```python
from build123d import *

# Parameters (mm, degrees)
F0_R      = 38.279248166
F2_R      = 18.7324901921
F5_R      = 38.2461043671
F3_FACE_R = 18.7324901921
F7_T      = -2.5


with BuildPart() as f3:
    # F0 (on Front) → F3 section 0
    with BuildSketch(Plane.XZ):
        Circle(F0_R)
    # F2 (on offset) → F3 section 1
    with BuildSketch(Plane.XZ.offset(100)):
        Circle(F2_R)
    loft()

    # F5 (on offset) → F6 section 0
    with BuildSketch(Plane.XZ.offset(200)):
        Circle(F5_R)
    # F3_face (on face) → F6 section 1
    with BuildSketch(Plane.XZ.offset(100)):
        Circle(F3_FACE_R)
    loft()

    # F7
    f7_openings = [f3.faces().sort_by_distance(p)[0] for p in [
        (0, -200, 0),
        (0, 0, 0),
    ]]
    offset(amount=F7_T, openings=f7_openings, kind=Kind.INTERSECTION)


solid = f3.part
```
Input: part model. Units: mm. Frame: model coordinates. A direction names the side the tool comes from. Give positions to 0.01 mm unless a question says otherwise; leave off trailing zeros. Loops run counter-clockwise (first coordinate to the right, second up) from the corner with the lowest first, then second, coordinate; pieces in that order, holes last. Notation, with made-up numbers: M 89,-18 L 106,-18 A14 cw 106,-2 Z; hole C -38,56 d4. An arc over 180 degrees is marked long. Answer as CSV lines item,"result". Start each with the question number.
1. Pull-direction query (Y, two-part tool) for faces 3 (the face through (34, 0, 12)), 4 (the face through (-22.513, -50.7, -17.262)), 5 (the face through (-20.48, -149.3, -15.7)); classes: released by +Y, released by -Y, zero draft, split by the parting line, or undercut.
2. Section A-A on x = 0. Return loops of the section in (y, z).
3. Reachability of faces 1 (the face through (27.043, -149.3, 8.516)), 2 (the face through (34, -200, 12)) from +Z, -Z, +X, -X, +Y, -Y: full face, straight path, thin tool, end or side. Return the list, or none.
4. Line query: L1, parallel to Z at x = -8.5, y = -29.5; L2, parallel to Z at x = 14, y = -154; L3, parallel to X at y = -111.5, z = -4.5. Output: solid intervals per line, ascending.
5. Section C-C on y = -79. Return loops of the section in (x, z), plus the area to 3 significant figures.
6. Pin query (flat end, axial travel): P1, Ø5, axis at y = -60.5, z = -18.5, coming from the -X side; P2, Ø10, axis at y = -32, z = -14, coming from the -X side; P3, Ø2, axis at y = -158, z = 9.5, coming from the +X side; P4, Ø1.5, axis at y = -141.5, z = 28.5, coming from the -X side (1 decimal). Return the tip coordinate at first contact, or that it passes through.
7. Section B-B on y = -142.5. Return loops of the section in (x, z), plus the area to 3 significant figures.
Computed values:
1,face 3,"released by +Y"
1,face 4,"undercut"
1,face 5,"released by -Y"
2,outline,"M -200,-38.25 L -100,-18.73 L 0,-38.28 L 0,-35.73 L -100,-16.19 L -200,-35.7 Z; M -200,35.7 L -100,16.19 L 0,35.73 L 0,38.28 L -100,18.73 L -200,38.25 Z"
3,face 1,"none"
3,face 2,"+Z, -Z, +X, -X, -Y"
4,L1,"z = -31.38 to -28.73, 28.73 to 31.38"
4,L2,"z = -25.7 to -22.76, 22.76 to 25.7"
4,L3,"x = -20.49 to -17.87, 17.87 to 20.49"
5,outline,"C 0,0 d45.67; hole C 0,0 d40.58"
5,area,"345 mm²"
6,P1,"stops at x = -21.16"
6,P2,"stops at x = -31.04"
6,P3,"stops at x = 28.89"
6,P4,"passes through"
7,outline,"C 0,0 d54.05; hole C 0,0 d48.96"
7,area,"412 mm²"
